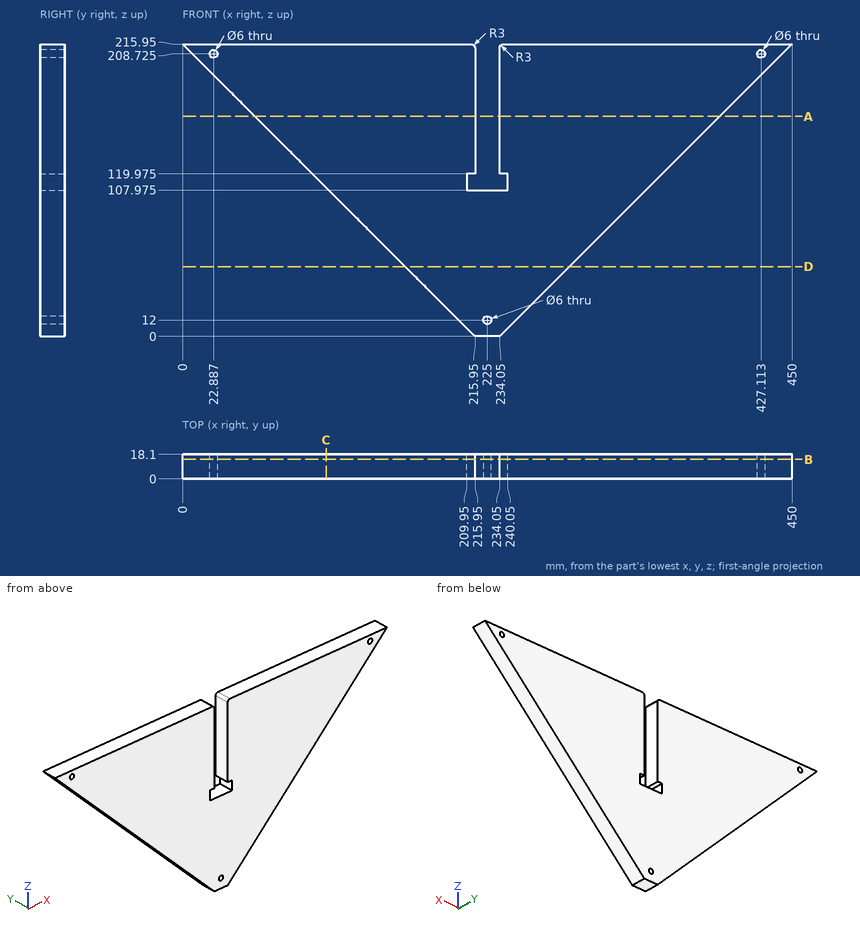
Can you work these out from the drawing? Everything is in mm from the part's minimum corner. Give positions to 0.01 mm unless a question says otherwise; leave off trailing zeros. Order: outer loops, then holes, each group sorted by start corner. A loop starts at its lowest first (then second) coordinate and runs counter-clockwise, first axis right, second up. Notation, with made-up numbers: M 29.5,87.25 L 83.5,87.25 A23 ccw 83.5,116.25 Z; hole C 79.5,-15 d5. An arc over 180 degrees is marked long. One line per question, with ' | ' between items.
1. I want a section at B-B (y = 14.5). Give the number of separate pieces and of enclosed holes in the cut face, and give its area (3 significant figures).
Results:
separate pieces: 1 | enclosed holes: 3 | area: 48,400 mm²
2. I want a section at C-C (x = 106). List the corners of the cut face in (y, z) for me, and give its area (3 significant figures).
Results:
outline: M 0,109.95 L 18.1,109.95 L 18.1,215.95 L 0,215.95 Z | area: 1,920 mm²
3. If I drill on line 1 (X direction, y = 10, z = 129.5); line 2 (X direction, y = 7.5, z = 12); line 3 (Z direction, x = 108, y = 12.25), over which ranges is the centre line in solid material (lowest first)?
Results:
line 1: 86.45 to 215.95, 234.05 to 363.55 | line 2: 203.95 to 222, 228 to 246.05 | line 3: 107.95 to 215.95
4. I'm going to push flat-ended pins straight in: pin 1 (10 mm diameter, centred on x = 295, z = 61.5, fed in from -Y); pin 2 (5.5 mm diameter, centred on x = 427.11, z = 208.72, fed in from +Y); pin 3 (1.5 mm diameter, centred on y = 4.5, z = 122.5, fed in from +X); pin 4 (5.5 mm diameter, centred on y = 9, z = 178, fed in from -X). Where does each tip first touch, or does it pass through?
Results:
pin 1: y = 0 | pin 2: through | pin 3: x = 357.3 | pin 4: x = 35.2
5. I want a section at D-D (z = 51.5). List the corners of the cut face in (x, y) for me, and give its area (3 significant figures).
Results:
outline: M 164.45,0 L 285.55,0 L 285.55,18.1 L 164.45,18.1 Z | area: 2,190 mm²
6. I want a section at A-A (z = 162.5). List the corners of the cut face in (x, y) for me, and give its area (3 significant figures).
Results:
outline: M 53.45,0 L 215.95,0 L 215.95,18.1 L 53.45,18.1 Z; M 234.05,0 L 396.55,0 L 396.55,18.1 L 234.05,18.1 Z | area: 5,880 mm²
